```python
from build123d import *

# Parameters (mm, degrees)
SKETCH1_W           = 25
SKETCH1_H           = 25
SKETCH1_W_2         = 21
SKETCH1_H_2         = 21
BOSS_EXTRUDE1_DEPTH = 275
SKETCH2_R           = 9.5
BOSS_EXTRUDE2_DEPTH = 6
CUT_EXTRUDE1_REACH  = 290.856
SKETCH3_R           = 5


with BuildPart() as part:
    # Sketch1 → Boss-Extrude1 (new body)
    with BuildSketch(Plane(origin=(0, 0, 0), x_dir=(1, 0, 0), z_dir=(0, 1, 0))):
        Rectangle(SKETCH1_W, SKETCH1_H)
        Rectangle(SKETCH1_W_2, SKETCH1_H_2, mode=Mode.SUBTRACT)
    extrude(amount=-BOSS_EXTRUDE1_DEPTH)

    # Sketch2 → Boss-Extrude2 (add)
    # profile 1 of 2: a face of its own
    with BuildSketch(Plane.XY.offset(12.5)):
        with BuildLine():
            Line((74.999020274, -17.752351341), (12.5, -5))
            Line((12.5, -5), (12.5, -55))
            Line((12.5, -55), (74.999020274, -42.247648659))
            ThreePointArc((74.999020274, -42.247648659), (85, -30), (74.999020274, -17.752351341))
        make_face()
        with Locations((72.5, -30)):
            Circle(SKETCH2_R, mode=Mode.SUBTRACT)
    # profile 2 of 2: a face of its own
    with BuildSketch(Plane.XY.offset(12.5)):
        with BuildLine():
            Line((89.528123749, -202.665628753), (12.5, -190))
            Line((12.5, -190), (12.5, -240))
            Line((12.5, -240), (89.528123749, -227.334371247))
            ThreePointArc((89.528123749, -227.334371247), (100, -215), (89.528123749, -202.665628753))
        make_face()
        with Locations((87.5, -215)):
            Circle(SKETCH2_R, mode=Mode.SUBTRACT)
    extrude(amount=-BOSS_EXTRUDE2_DEPTH)

    # Cut-Extrude1: up to this face of the body (flat: up to its plane)
    cut_extrude1_end = Plane(part.part.faces().sort_by_distance((-12.5, -137.5, 0))[0])
    # Sketch3 → Cut-Extrude1 (cut, up to the picked face)
    with BuildSketch(Plane(origin=(12.5, 0, 0), x_dir=(0, 0, -1), z_dir=(1, 0, 0)), mode=Mode.PRIVATE) as cut_extrude1_sk1:
        with Locations((-4.5, -115)):
            Circle(SKETCH3_R)
    cut_extrude1_tool1 = split(extrude(cut_extrude1_sk1.sketch, amount=-CUT_EXTRUDE1_REACH, mode=Mode.PRIVATE), bisect_by=cut_extrude1_end, keep=Keep.BOTH, mode=Mode.PRIVATE)
    # Sketch3 → Cut-Extrude1 (cut, up to the picked face)
    with BuildSketch(Plane(origin=(12.5, 0, 0), x_dir=(0, 0, -1), z_dir=(1, 0, 0)), mode=Mode.PRIVATE) as cut_extrude1_sk2:
        with Locations((-4.5, -255)):
            Circle(SKETCH3_R)
    cut_extrude1_tool2 = split(extrude(cut_extrude1_sk2.sketch, amount=-CUT_EXTRUDE1_REACH, mode=Mode.PRIVATE), bisect_by=cut_extrude1_end, keep=Keep.BOTH, mode=Mode.PRIVATE)
    add(cut_extrude1_tool1.solids().sort_by(Axis((12.5, -115, 4.5), (-1, 0, 0)))[0], mode=Mode.SUBTRACT)
    add(cut_extrude1_tool2.solids().sort_by(Axis((12.5, -255, 4.5), (-1, 0, 0)))[0], mode=Mode.SUBTRACT)


solid = part.part
```
Here's how the part is built. I have some questions about the finished solid (model axes, mm). A direction names the side the tool comes from. Coordinates: 2 decimals unless noted, no trailing zeros. Loops run counter-clockwise (first coordinate to the right, second up) from the corner with the lowest first, then second, coordinate; pieces in that order, holes last. Notation, with made-up numbers: M 79.5,50 L 119.5,50 A6 cw 119.5,55 Z; hole C -39.75,34 d2. An arc over 180 degrees is marked long. One line per item, written item: value.
1. Please list where these lines run through material, in increasing order: probe 1 along Y at (x, z) = (-11.9, 4.5); probe 2 along X at (y, z) = (-158.5, 3); probe 3 along Y at (x, z) = (72.5, 10.05).
Geometry says:
probe 1: y = -275 to -260, -250 to -120, -110 to 0
probe 2: x = -12.5 to -10.5, 10.5 to 12.5
probe 3: y = -230.13 to -199.87, -42.76 to -39.5, -20.5 to -17.24
2. Thinking about a two-plate mould opening in Z: for faces 4 (the cylindrical face through (85.441, -224.274, 9.542)), 5 (the flat face through (0, -136, 10.5)), 6 (the flat face through (5, -136, 12.5)), which applies, +Z half, -Z half, draft (parallel to the pull), parting line (faces both ways), or undercut?
Geometry says:
face 4: draft
face 5: undercut
face 6: +Z half
3. On a 3-axis mill with a long thin cutter (end or side, diameter ignored), from which of +Z, -Z, +X, -X, +Y, -Y can I reach the whole of each face in a straight line? I mean faces 1 (the flat face through (40, -30, 6.5)), 2 (the flat face through (-10.5, -136, 0)), 3 (the flat face through (43.312, -48.713, 9.542)). Say none if no direction works.
Geometry says:
face 1: -Z, +X, +Y, -Y
face 2: +Y, -Y
face 3: +Z, -Z, +X
4. Imagine slicing it at D-D (z = -4.5). List the corners of the cut face in (x, y) for me.
Geometry says:
outline: M -12.5,-275 L -10.5,-275 L -10.5,0 L -12.5,0 Z; M 10.5,-275 L 12.5,-275 L 12.5,0 L 10.5,0 Z
5. Imagine slicing it at B-B (x = 6). List the corners of the cut face in (y, z) for me.
Geometry says:
outline: M -275,-12.5 L 0,-12.5 L 0,-10.5 L -275,-10.5 Z; M -275,10.5 L 0,10.5 L 0,12.5 L -275,12.5 Z
6. Will these pins go through, and if not, where does the flat tip stop? pin 1 Ø15 at (x, y) = (44, -204.5) entering from -Z; pin 2 Ø9 at (y, z) = (-115, 4.5) entering from +X; pin 3 Ø6.5 at (y, z) = (-164, 0) entering from +X; pin 4 Ø12 at (x, z) = (27, 9.5) entering from -Y.
Geometry says:
pin 1: stops at z = 6.5
pin 2: passes through
pin 3: stops at x = 12.5
pin 4: stops at y = -238.6
7. Imagine slicing it at A-A (y = -30). List the corners of the cut face in (x, z) for me, and give its area (3 significant figures).
Geometry says:
outline: M -12.5,-12.5 L 12.5,-12.5 L 12.5,6.5 L 63,6.5 L 63,12.5 L -12.5,12.5 Z; M 82,6.5 L 85,6.5 L 85,12.5 L 82,12.5 Z; hole M -10.5,-10.5 L 10.5,-10.5 L 10.5,10.5 L -10.5,10.5 Z
area: 505 mm2
8. Imagine slicing it at C-C (y = -255). List the corners of the cut face in (x, z) for me, and give its area (3 significant figures).
Geometry says:
outline: M -12.5,-12.5 L 12.5,-12.5 L 12.5,-0.5 L 10.5,-0.5 L 10.5,-10.5 L -10.5,-10.5 L -10.5,-0.5 L -12.5,-0.5 Z; M -12.5,9.5 L -10.5,9.5 L -10.5,10.5 L 10.5,10.5 L 10.5,9.5 L 12.5,9.5 L 12.5,12.5 L -12.5,12.5 Z
area: 144 mm2
